Check sheet for the modelled part. Datum: model origin and axes. Units: mm. Round coordinates to 2 decimals unless told otherwise and drop trailing zeros. Loops run counter-clockwise (first coordinate to the right, second up) from the corner with the lowest first, then second, coordinate; pieces in that order, holes last. Notation, with made-up numbers: (22, 65) -> (58, 65) arc R19 cw to (58, 69) -> close; hole circle Ø3 at (50.25, 79). An arc over 180 degrees is marked (long way). One line per item, written item: value. Start each with the question number.
1. Cross-section at D-D on x = 4. Record the cut outline in (y, z) (3 decimals), then the cut area to 3 significant figures.
2. Material ranges on L1, parallel to X at y = 11.5, z = 2.6; L2, parallel to X at y = 30.5, z = 1.35, recorded low to high.
3. Go/stop test with a flat-tipped pin: pin 1 (1.5 mm diameter, centred on x = 17, z = 1.5, fed in from -Y). Record where the tip stops, or that it passes through.
4. Cross-section at C-C on x = 24.5. Record the cut outline in (y, z) (3 decimals).
5. Cross-section at B-B on y = 27.5. Record the cut outline in (x, z) (3 decimals).
6. Cross-section at A-A on x = 18. Record the cut outline in (y, z) (3 decimals), then the cut area to 3 significant figures.
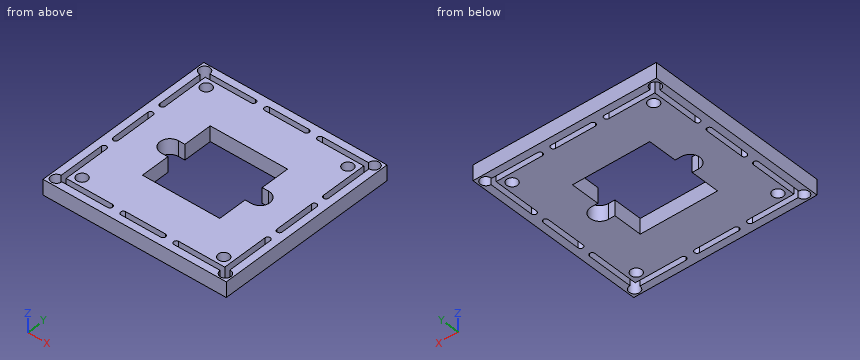
from build123d import *

# Parameters (mm, degrees)
SKETCH1_W           = 37.9349
SKETCH1_H           = 37.9349
BOSS_EXTRUDE1_DEPTH = 3.175
SKETCH9_R           = 1.1176
CUT_EXTRUDE2_DEPTH  = 3.175
SKETCH10_W          = 16.002
SKETCH10_H          = 16.002
CUT_EXTRUDE3_DEPTH  = 3.175
CUT_EXTRUDE4_DEPTH  = 3.175


with BuildPart() as part:
    # Sketch1 → Boss-Extrude1 (new body)
    with BuildSketch(Plane.XY):
        with Locations((18.96745, 18.96745)):
            Rectangle(SKETCH1_W, SKETCH1_H)
    extrude(amount=BOSS_EXTRUDE1_DEPTH)

    # Sketch9 → Cut-Extrude2 (cut)
    with BuildSketch(Plane.XY.offset(3.175)):
        with Locations((33.62325, 33.62325)):
            Circle(SKETCH9_R)
        with Locations((4.31165, 33.62325)):
            Circle(SKETCH9_R)
        with Locations((4.31165, 4.31165)):
            Circle(SKETCH9_R)
        with Locations((33.62325, 4.31165)):
            Circle(SKETCH9_R)
        with BuildLine():
            Line((35.385619933, 12.100169933), (35.385619933, 2.549280067))
            Line((35.385619933, 2.549280067), (25.834730067, 2.549280067))
            ThreePointArc((25.834730067, 2.549280067), (25.2984, 2.01295), (25.834730067, 1.476619933))
            Line((25.834730067, 1.476619933), (35.385619933, 1.476619933))
            ThreePointArc((35.385619933, 1.476619933), (37.303202335, 0.631697665), (36.458280067, 2.549280067))
            Line((36.458280067, 2.549280067), (36.458280067, 12.100169933))
            ThreePointArc((36.458280067, 12.100169933), (35.92195, 12.6365), (35.385619933, 12.100169933))
        make_face()
        with BuildLine():
            Line((35.385619933, 36.458280067), (25.834730067, 36.458280067))
            ThreePointArc((25.834730067, 36.458280067), (25.2984, 35.92195), (25.834730067, 35.385619933))
            Line((25.834730067, 35.385619933), (35.385619933, 35.385619933))
            Line((35.385619933, 35.385619933), (35.385619933, 25.834730067))
            ThreePointArc((35.385619933, 25.834730067), (35.92195, 25.2984), (36.458280067, 25.834730067))
            Line((36.458280067, 25.834730067), (36.458280067, 35.385619933))
            ThreePointArc((36.458280067, 35.385619933), (37.303202335, 37.303202335), (35.385619933, 36.458280067))
        make_face()
        with BuildLine():
            Line((12.048880067, 36.458280067), (2.549280067, 36.458280067))
            ThreePointArc((2.549280067, 36.458280067), (0.631697665, 37.303202335), (1.476619933, 35.385619933))
            Line((1.476619933, 35.385619933), (1.476619933, 25.886019933))
            ThreePointArc((1.476619933, 25.886019933), (2.01295, 25.349689867), (2.549280067, 25.886019933))
            Line((2.549280067, 25.886019933), (2.549280067, 35.385619933))
            Line((2.549280067, 35.385619933), (12.048880067, 35.385619933))
            ThreePointArc((12.048880067, 35.385619933), (12.585210133, 35.92195), (12.048880067, 36.458280067))
        make_face()
        with BuildLine():
            Line((23.06955, 36.458280067), (14.86535, 36.458280067))
            ThreePointArc((14.86535, 36.458280067), (14.329019933, 35.92195), (14.86535, 35.385619933))
            Line((14.86535, 35.385619933), (23.06955, 35.385619933))
            ThreePointArc((23.06955, 35.385619933), (23.605880067, 35.92195), (23.06955, 36.458280067))
        make_face()
        with BuildLine():
            Line((2.549280067, 23.06955), (2.549280067, 14.86535))
            ThreePointArc((2.549280067, 14.86535), (2.01295, 14.329019933), (1.476619933, 14.86535))
            Line((1.476619933, 14.86535), (1.476619933, 23.06955))
            ThreePointArc((1.476619933, 23.06955), (2.01295, 23.605880067), (2.549280067, 23.06955))
        make_face()
        with BuildLine():
            Line((36.458280067, 23.06955), (36.458280067, 14.86535))
            ThreePointArc((36.458280067, 14.86535), (35.92195, 14.329019933), (35.385619933, 14.86535))
            Line((35.385619933, 14.86535), (35.385619933, 23.06955))
            ThreePointArc((35.385619933, 23.06955), (35.92195, 23.605880067), (36.458280067, 23.06955))
        make_face()
        with BuildLine():
            Line((23.06955, 2.549280067), (14.86535, 2.549280067))
            ThreePointArc((14.86535, 2.549280067), (14.329019933, 2.01295), (14.86535, 1.476619933))
            Line((14.86535, 1.476619933), (23.06955, 1.476619933))
            ThreePointArc((23.06955, 1.476619933), (23.605880067, 2.01295), (23.06955, 2.549280067))
        make_face()
        with BuildLine():
            Line((2.549280067, 12.100169933), (2.549280067, 2.549280067))
            Line((2.549280067, 2.549280067), (12.100169933, 2.549280067))
            ThreePointArc((12.100169933, 2.549280067), (12.6365, 2.01295), (12.100169933, 1.476619933))
            Line((12.100169933, 1.476619933), (2.600569933, 1.476619933))
            ThreePointArc((2.600569933, 1.476619933), (0.681867267, 0.681867267), (1.476619933, 2.600569933))
            Line((1.476619933, 2.600569933), (1.476619933, 12.100169933))
            ThreePointArc((1.476619933, 12.100169933), (2.01295, 12.6365), (2.549280067, 12.100169933))
        make_face()
    extrude(amount=-CUT_EXTRUDE2_DEPTH, mode=Mode.SUBTRACT)

    # Sketch10 → Cut-Extrude3 (cut)
    with BuildSketch(Plane(origin=(0, 0, 0), x_dir=(-1, 0, 0), z_dir=(0, 0, -1))):
        with Locations((-18.96745, 18.96745)):
            Rectangle(SKETCH10_W, SKETCH10_H)
    extrude(amount=-CUT_EXTRUDE3_DEPTH, mode=Mode.SUBTRACT)

    # Sketch11 → Cut-Extrude4 (cut)
    with BuildSketch(Plane(origin=(0, 0, 0), x_dir=(-1, 0, 0), z_dir=(0, 0, -1))):
        with BuildLine():
            Line((-10.96645, 16.9545), (-9.62787, 16.9545))
            ThreePointArc((-9.62787, 16.9545), (-7.61492, 18.96745), (-9.62787, 20.9804))
            Line((-9.62787, 20.9804), (-10.96645, 20.9804))
            Line((-10.96645, 20.9804), (-10.96645, 16.9545))
        make_face()
        with BuildLine():
            Line((-28.30703, 20.9804), (-26.96845, 20.9804))
            Line((-26.96845, 20.9804), (-26.96845, 16.9545))
            Line((-26.96845, 16.9545), (-28.30703, 16.9545))
            ThreePointArc((-28.30703, 16.9545), (-30.31998, 18.96745), (-28.30703, 20.9804))
        make_face()
    extrude(amount=-CUT_EXTRUDE4_DEPTH, mode=Mode.SUBTRACT)


solid = part.part
Taken from the geometry:
1. outline: (0, 0) -> (1.477, 0) -> (1.477, 3.175) -> (0, 3.175) -> close; (2.549, 0) -> (3.238, 0) -> (3.238, 3.175) -> (2.549, 3.175) -> close; (5.385, 0) -> (32.55, 0) -> (32.55, 3.175) -> (5.385, 3.175) -> close; (34.697, 0) -> (35.386, 0) -> (35.386, 3.175) -> (34.697, 3.175) -> close; (36.458, 0) -> (37.935, 0) -> (37.935, 3.175) -> (36.458, 3.175) -> close
1. area: 100 mm2
2. L1: x = 0 to 1.48, 2.55 to 10.97, 26.97 to 35.39, 36.46 to 37.93
2. L2: x = 0 to 1.48, 2.55 to 35.39, 36.46 to 37.93
3. pin 1: stops at y = 0
4. outline: (0, 0) -> (10.966, 0) -> (10.966, 3.175) -> (0, 3.175) -> close; (26.968, 0) -> (37.935, 0) -> (37.935, 3.175) -> (26.968, 3.175) -> close
5. outline: (0, 0) -> (1.477, 0) -> (1.477, 3.175) -> (0, 3.175) -> close; (2.549, 0) -> (35.386, 0) -> (35.386, 3.175) -> (2.549, 3.175) -> close; (36.458, 0) -> (37.935, 0) -> (37.935, 3.175) -> (36.458, 3.175) -> close
6. outline: (0, 0) -> (1.477, 0) -> (1.477, 3.175) -> (0, 3.175) -> close; (2.549, 0) -> (10.966, 0) -> (10.966, 3.175) -> (2.549, 3.175) -> close; (26.968, 0) -> (35.386, 0) -> (35.386, 3.175) -> (26.968, 3.175) -> close; (36.458, 0) -> (37.935, 0) -> (37.935, 3.175) -> (36.458, 3.175) -> close
6. area: 62.8 mm2
